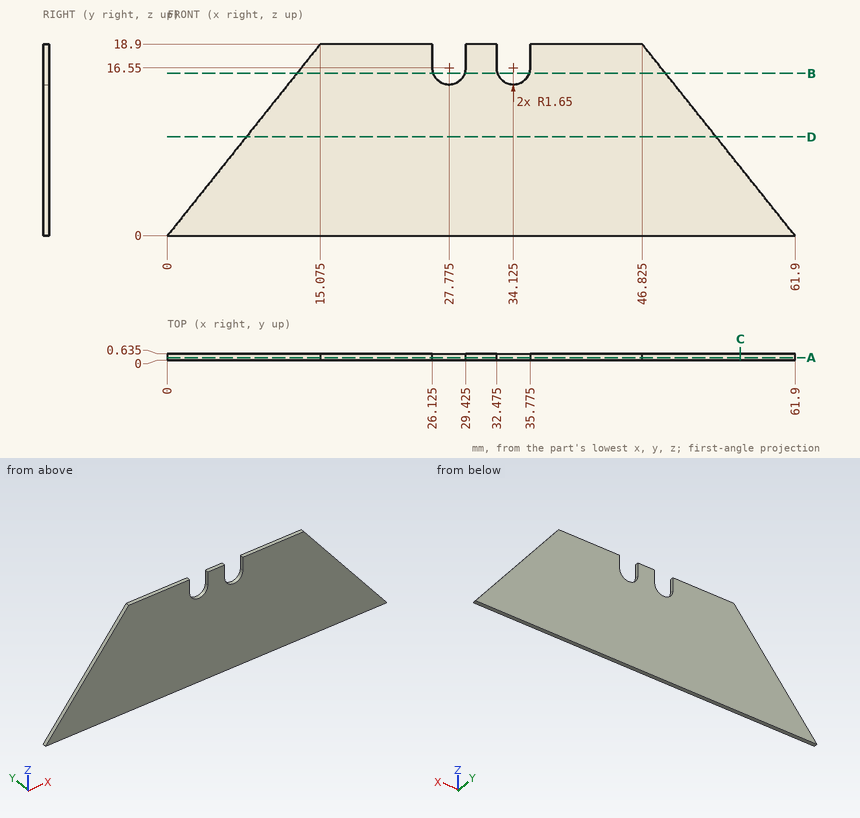
Drawing for the job (mm, zero at the part's lowest x, y, z). Round coordinates to 2 decimals unless told otherwise and drop trailing zeros. Loops run counter-clockwise (first coordinate to the right, second up) from the corner with the lowest first, then second, coordinate; pieces in that order, holes last. Notation, with made-up numbers: (12, -26.75) -> (38, -26.75) arc R32 ccw to (38, 10.25) -> close; hole circle Ø1 at (42, -17). An arc over 180 degrees is marked (long way). Answer in a Markdown table with one row per item.
Item 1: Saw through at C-C (x = 56.5). Write the cut outline in (y, z) (3 decimals), and give its area (3 significant figures).
Answers below:
| item | result |
|---|---|
| outline | (0, 0) -> (0.635, 0) -> (0.635, 6.77) -> (0, 6.77) -> close |
| area | 4.30 mm² |
Item 2: Saw through at A-A (y = 0.25). Write the cut outline in (x, z) (3 decimals), and give its area (3 significant figures).
Answers below:
| item | result |
|---|---|
| outline | (0, 0) -> (61.9, 0) -> (46.825, 18.9) -> (35.775, 18.9) -> (35.775, 16.55) arc R1.65 cw to (32.475, 16.55) -> (32.475, 18.9) -> (29.425, 18.9) -> (29.425, 16.55) arc R1.65 cw to (26.125, 16.55) -> (26.125, 18.9) -> (15.075, 18.9) -> close |
| area | 861 mm² |
Item 3: Drill centre lines: L1, parallel to X at y = 0.45, z = 13.75; L2, parallel to Z at x = 35, y = 0.5; L3, parallel to X at y = 0.2, z = 11. Where is each one in solid material? Low to high. Write a range as [from, to].
Answers below:
| item | result |
|---|---|
| L1 | x = [10.97, 50.93] |
| L2 | z = [0, 15.15] |
| L3 | x = [8.77, 53.13] |
Item 4: Saw through at D-D (z = 9.75). Write the cut outline in (x, y) (3 decimals), and give its area (3 significant figures).
Answers below:
| item | result |
|---|---|
| outline | (7.777, 0) -> (54.123, 0) -> (54.123, 0.635) -> (7.777, 0.635) -> close |
| area | 29.4 mm² |
Item 5: Saw through at B-B (z = 16). Write the cut outline in (x, y) (3 decimals), and give its area (3 significant figures).
Answers below:
| item | result |
|---|---|
| outline | (12.762, 0) -> (26.219, 0) -> (26.219, 0.635) -> (12.762, 0.635) -> close; (29.331, 0) -> (32.569, 0) -> (32.569, 0.635) -> (29.331, 0.635) -> close; (35.681, 0) -> (49.138, 0) -> (49.138, 0.635) -> (35.681, 0.635) -> close |
| area | 19.1 mm² |
